from build123d import *

# Parameters (mm, degrees)
F0_W      = 254
F0_H      = 254
F1_DEPTH  = 6.35
F4_DEPTH  = 25.4
F5_W      = 6.35
F5_H      = 127
F6_DEPTH  = 25.4
F7_W      = 165.1
F7_H      = 6.35
F8_DEPTH  = 25.4
F9_R      = 6.35
F10_DEPTH = 7.62
F11_R     = 3.81
F14_DEPTH = 7.62
F13_R     = 1.27
F15_DEPTH = 25.4
F2_W      = 6.35
F2_H      = 127
F16_DEPTH = 25.4


with BuildPart() as f1:
    # F0 (on Top) → F1 (new body)
    with BuildSketch(Plane.XY):
        Rectangle(F0_W, F0_H)
    extrude(amount=F1_DEPTH)

    # F3 (on face) → F4 (cut)
    with BuildSketch(Plane.XY.offset(6.35)):
        Polygon((114.3, -53.975), (-50.8, -53.975), (-50.8, -60.325), (114.3, -60.325), (114.3, -57.15), (114.3, -56.917642), align=None)
    extrude(amount=-F4_DEPTH, mode=Mode.SUBTRACT)

    # F5 (on face) → F6 (cut)
    with BuildSketch(Plane.XY.offset(6.35)):
        with Locations((47.625, -57.15)):
            Rectangle(F5_W, F5_H)
    extrude(amount=-F6_DEPTH, mode=Mode.SUBTRACT)

    # F7 (on face) → F8 (cut)
    with BuildSketch(Plane.XY.offset(6.35)):
        with Locations((-31.75, 57.15)):
            Rectangle(F7_W, F7_H)
    extrude(amount=-F8_DEPTH, mode=Mode.SUBTRACT)

    # F9 (on face) → F10 (join)
    with BuildSketch(Plane(origin=(0, 0, 0), x_dir=(1, 0, 0), z_dir=(0, 0, -1))):
        Circle(F9_R)
    extrude(amount=F10_DEPTH)

    # F11 (on face) → F14 (cut)
    with BuildSketch(Plane(origin=(0, 0, -7.62), x_dir=(1, 0, 0), z_dir=(0, 0, -1))):
        Circle(F11_R)
    extrude(amount=-F14_DEPTH, mode=Mode.SUBTRACT)

    # F13 (on offset) → F15 (cut)
    with BuildSketch(Plane.XZ.offset(-12.7)):
        with Locations((0, -2.54)):
            Circle(F13_R)
    extrude(amount=F15_DEPTH, mode=Mode.SUBTRACT)

    # F2 (on face) → F16 (cut)
    with BuildSketch(Plane.XY.offset(6.35)):
        with Locations((-47.625, 57.15)):
            Rectangle(F2_W, F2_H)
    extrude(amount=-F16_DEPTH, mode=Mode.SUBTRACT)


solid = f1.part
The listing builds one solid part. Answer for the finished solid, in the listing's coordinates (mm). A direction names the side the tool comes from. Give positions to 0.01 mm unless a question says otherwise; leave off trailing zeros. Write each loop counter-clockwise with the first axis right and the second up, starting at its lowest first coordinate (ties: lowest second). Pieces come first, ordered by that corner, then holes.
1) Find the intervals of material crossed by L1, parallel to Y at x = 0, z = 0.75 (3 decimals); L2, parallel to X at y = 60, z = 5; L3, parallel to Y at x = 0, z = -5.75, in increasing order.
2) Section A-A (y = -70.5) is taken. Write down the section's boundary in (x, z).
3) For a pull along X with two mould halves and no side action, classify faces 1 (the face through (-50.8, -57, 3)), 2 (the face through (-2, -127, 3)), 3 (the face through (-127, -2, 3)) as pulls with the +X half, pulls with the -X half, needs draft (parallel to the pull), parting line crosses it, or undercut.
4) A tool of negligible diameter and unlimited length cuts with its end or side. For faces 4 (the face through (-2, 127, 3)), 5 (the face through (3.52, 1.46, -3.86)), 6 (the face through (-44.45, 90, 3)), from which of +Z, -Z, +X, -X, +Y, -Y can it reach the whole face along a straight path? Write none if from no direction.
5) Section D-D (z = 3.75) is taken. Write down the section's boundary in (x, y) (3 decimals).
6) Section C-C (y = 0) is taken. Write down the section's boundary in (x, z), and give its area (3 significant figures).
7) Given P1, Ø1.5, axis at x = 5, z = -5.5, coming from the -Y side; P2, Ø6, axis at x = 1, y = -1, coming from the -Z side; P3, Ø4, axis at x = 36, y = -27, coming from the -Z side, each flat-ended and moving along its own axis, determine where each tip first touches the part or whether it passes through.
8) Section B-B (x = -70.5) is taken. Write down the section's boundary in (y, z) (3 decimals), and give its area (3 significant figures).
Response:
1. L1: y = -127 to -60.325, -53.975 to 53.975, 60.325 to 127
1. L2: x = -127 to -114.3, 50.8 to 127
1. L3: y = -6.35 to -3.81, 3.81 to 6.35
2. outline: (-127, 0) - (44.45, 0) - (44.45, 6.35) - (-127, 6.35) - close; (50.8, 0) - (127, 0) - (127, 6.35) - (50.8, 6.35) - close
3. face 1: undercut
3. face 2: needs draft
3. face 3: pulls with the -X half
4. face 4: +Z, -Z, +X, -X, +Y
4. face 5: -Z
4. face 6: +Z, -Z
5. outline: (-127, -127) - (127, -127) - (127, 127) - (-127, 127) - close; hole (-114.3, 53.975) - (-50.8, 53.975) - (-50.8, -6.35) - (-44.45, -6.35) - (-44.45, 53.975) - (50.8, 53.975) - (50.8, 60.325) - (-44.45, 60.325) - (-44.45, 120.65) - (-50.8, 120.65) - (-50.8, 60.325) - (-114.3, 60.325) - close; hole (-50.8, -60.325) - (44.45, -60.325) - (44.45, -120.65) - (50.8, -120.65) - (50.8, -60.325) - (114.3, -60.325) - (114.3, -53.975) - (50.8, -53.975) - (50.8, 6.35) - (44.45, 6.35) - (44.45, -53.975) - (-50.8, -53.975) - close
6. outline: (-127, 0) - (-50.8, 0) - (-50.8, 6.35) - (-127, 6.35) - close; (-44.45, 0) - (-6.35, 0) - (-6.35, -7.62) - (-3.81, -7.62) - (-3.81, 0) - (3.81, 0) - (3.81, -7.62) - (6.35, -7.62) - (6.35, 0) - (44.45, 0) - (44.45, 6.35) - (-44.45, 6.35) - close; (50.8, 0) - (127, 0) - (127, 6.35) - (50.8, 6.35) - close
6. area: 1,570 mm2
7. P1: stops at y = -4.72
7. P2: stops at z = -7.62
7. P3: stops at z = 0
8. outline: (-127, 0) - (53.975, 0) - (53.975, 6.35) - (-127, 6.35) - close; (60.325, 0) - (127, 0) - (127, 6.35) - (60.325, 6.35) - close
8. area: 1,570 mm2
